from build123d import *

# Parameters (mm, degrees)
SKETCH1_R                      = 15.35
BOSS_EXTRUDE1_DEPTH            = 2.71
SKETCH2_R                      = 2.685
BOSS_EXTRUDE2_DEPTH            = 1.2
DOME1_FACE_RADIUS              = 2.685
DOME1_HEIGHT                   = 0.6
CIRPATTERN1_COUNT              = 3
CIRPATTERN1_COPY_1_FACE_RADIUS = 2.685
CIRPATTERN1_COPY_1_HEIGHT      = 0.6
CIRPATTERN1_COPY_2_FACE_RADIUS = 2.685
CIRPATTERN1_COPY_2_HEIGHT      = 0.6
BOSS_EXTRUDE3_START            = 2.55
SKETCH3_W                      = 5.5
SKETCH3_H                      = 4.2
SKETCH3_W_2                    = 1.5
SKETCH3_H_2                    = 2.8
BOSS_EXTRUDE3_DEPTH            = 2.55
SKETCH4_W                      = 5.5
SKETCH4_H                      = 4.2
BOSS_EXTRUDE4_DEPTH            = 1.44
CHIP_DEPTH                     = 1.7018


with BuildPart() as part:
    # Sketch1 → Boss-Extrude1 (new body)
    with BuildSketch(Plane(origin=(0, 0, 0), x_dir=(1, 0, 0), z_dir=(0, 1, 0))):
        with Locations(Location((0, 0, 0), (0, 0, 270))):
            Circle(SKETCH1_R)
    extrude(amount=BOSS_EXTRUDE1_DEPTH)

    # Sketch2 → Boss-Extrude2 (add)
    with BuildSketch(Plane(origin=(0, 2.71, 0), x_dir=(-1, 0, 0), z_dir=(0, 1, 0))):
        with Locations(Location((-5.5, 9.526279442, 0), (0, 0, 90))):
            Circle(SKETCH2_R)
    boss_extrude2 = extrude(amount=BOSS_EXTRUDE2_DEPTH)

    # Dome1: a dome of height H over a round flat face of radius A is a cap of a sphere of radius (A * A + H * H) / (2 * H)
    dome1_r = (DOME1_FACE_RADIUS * DOME1_FACE_RADIUS + DOME1_HEIGHT * DOME1_HEIGHT) / (2 * DOME1_HEIGHT)
    dome1_base = Plane((5.5, 3.91, 9.526279442), z_dir=(0, 1, 0))
    with Locations(dome1_base.offset(DOME1_HEIGHT - dome1_r)):
        dome1_ball = Sphere(dome1_r, mode=Mode.PRIVATE)
    add(split(dome1_ball, bisect_by=dome1_base, keep=Keep.TOP, mode=Mode.PRIVATE))

    # CirPattern1: Boss-Extrude2 ×3 about axis
    cirpattern1_axis = Axis((0, 0, 0), (0, 1, 0))
    for i in range(1, CIRPATTERN1_COUNT):
        add(boss_extrude2.rotate(cirpattern1_axis, i * 360 / CIRPATTERN1_COUNT))

    # CirPattern1 copy 1: a dome of height H over a round flat face of radius A is a cap of a sphere of radius (A * A + H * H) / (2 * H)
    cirpattern1_copy_1_r = (CIRPATTERN1_COPY_1_FACE_RADIUS * CIRPATTERN1_COPY_1_FACE_RADIUS + CIRPATTERN1_COPY_1_HEIGHT * CIRPATTERN1_COPY_1_HEIGHT) / (2 * CIRPATTERN1_COPY_1_HEIGHT)
    cirpattern1_copy_1_base = Plane((5.5, 3.91, -9.526279442), z_dir=(0, 1, 0))
    with Locations(cirpattern1_copy_1_base.offset(CIRPATTERN1_COPY_1_HEIGHT - cirpattern1_copy_1_r)):
        cirpattern1_copy_1_ball = Sphere(cirpattern1_copy_1_r, mode=Mode.PRIVATE)
    add(split(cirpattern1_copy_1_ball, bisect_by=cirpattern1_copy_1_base, keep=Keep.TOP, mode=Mode.PRIVATE))

    # CirPattern1 copy 2: a dome of height H over a round flat face of radius A is a cap of a sphere of radius (A * A + H * H) / (2 * H)
    cirpattern1_copy_2_r = (CIRPATTERN1_COPY_2_FACE_RADIUS * CIRPATTERN1_COPY_2_FACE_RADIUS + CIRPATTERN1_COPY_2_HEIGHT * CIRPATTERN1_COPY_2_HEIGHT) / (2 * CIRPATTERN1_COPY_2_HEIGHT)
    cirpattern1_copy_2_base = Plane((-11, 3.91, 0), z_dir=(0, 1, 0))
    with Locations(cirpattern1_copy_2_base.offset(CIRPATTERN1_COPY_2_HEIGHT - cirpattern1_copy_2_r)):
        cirpattern1_copy_2_ball = Sphere(cirpattern1_copy_2_r, mode=Mode.PRIVATE)
    add(split(cirpattern1_copy_2_ball, bisect_by=cirpattern1_copy_2_base, keep=Keep.TOP, mode=Mode.PRIVATE))

    # Sketch3 → Boss-Extrude3 (add)
    with BuildSketch(Plane.XZ.offset(BOSS_EXTRUDE3_START)):
        with Locations((0, 13.05)):
            Rectangle(SKETCH3_W, SKETCH3_H)
        with Locations((0, -13.05)):
            Rectangle(SKETCH3_W, SKETCH3_H)
        with Locations((3.5, 13.05)):
            Rectangle(SKETCH3_W_2, SKETCH3_H_2)
        with Locations((-3.5, 13.05)):
            Rectangle(SKETCH3_W_2, SKETCH3_H_2)
        with Locations((3.5, -13.05)):
            Rectangle(SKETCH3_W_2, SKETCH3_H_2)
        with Locations((-3.5, -13.05)):
            Rectangle(SKETCH3_W_2, SKETCH3_H_2)
        with BuildLine():
            Line((2.75, 15.101655538), (2.75, 15.15))
            Line((2.75, 15.15), (2.469817807, 15.15))
            ThreePointArc((2.469817807, 15.15), (2.610020839, 15.126476497), (2.75, 15.101655538))
        make_face()
        with BuildLine():
            ThreePointArc((-2.75, 15.101655538), (-2.610020839, 15.126476497), (-2.469817807, 15.15))
            Line((-2.469817807, 15.15), (-2.75, 15.15))
            Line((-2.75, 15.15), (-2.75, 15.101655538))
        make_face()
        with BuildLine():
            ThreePointArc((-2.469817807, -15.15), (-2.610020839, -15.126476497), (-2.75, -15.101655538))
            Line((-2.75, -15.101655538), (-2.75, -15.15))
            Line((-2.75, -15.15), (-2.469817807, -15.15))
        make_face()
        with BuildLine():
            Line((2.75, -15.15), (2.75, -15.101655538))
            ThreePointArc((2.75, -15.101655538), (2.610020839, -15.126476497), (2.469817807, -15.15))
            Line((2.469817807, -15.15), (2.75, -15.15))
        make_face()
    extrude(amount=-BOSS_EXTRUDE3_DEPTH)

    # Sketch4 → Boss-Extrude4 (add)
    with BuildSketch(Plane.XZ.offset(2.55)):
        Polygon((-2.75, 10.95), (2.75, 10.95), (2.75, 11.65), (2.75, 14.45), (2.75, 15.15), (-2.75, 15.15), (-2.75, 14.45), (-2.75, 11.65), align=None)
        with Locations((0, -13.05)):
            Rectangle(SKETCH4_W, SKETCH4_H)
    extrude(amount=BOSS_EXTRUDE4_DEPTH)

    # Sketch5 → Chip (add)
    with BuildSketch(Plane.XZ):
        Polygon((-5.1644, -9.425953844), (-2.016601499, -2.878979584), (-8.014179317, 0.004667994), (-11.161977818, -6.542306266), align=None)
    extrude(amount=CHIP_DEPTH)


solid = part.part
Geometry check sheet. Reference: the model listing, model coordinates, mm. A direction names the side the tool comes from. Give positions to 0.01 mm unless a question says otherwise; leave off trailing zeros. Order: outer loops, then holes, each group sorted by start corner. A loop starts at its lowest first (then second) coordinate and runs counter-clockwise, first axis right, second up. Notation, with made-up numbers: (24, 82) - (50, 82) arc R6 cw to (50, 89) - close; hole circle Ø8 at (54, -21). An arc over 180 degrees is marked (long way). Answer as a JSON object with one key per item and string values.
(1) Cross-section at B-B (z = -10.5). Record the cut outline in (x, y), then the cut area to 3 significant figures.
Report:
{"outline": "(-11.2, 0) - (11.2, 0) - (11.2, 2.71) - (8, 2.71) - (8, 3.91) arc R6.23 ccw to (3, 3.91) - (3, 2.71) - (-11.2, 2.71) - close", "area": "68.5 mm^2"}
(2) Depth check by flat-ended pin: pin 1 Ø1.3 at (y, z) = (-1.5, -13.5) entering from -X; pin 2 Ø5 at (x, z) = (10.5, 4) entering from -Y; pin 3 Ø1 at (x, z) = (-7.5, -7.5) entering from -Y; pin 4 Ø1.5 at (x, y) = (-2, 3.5) entering from +Z. Enter the tip coordinate at first touch or a pass-through.
Report:
{"pin 1": "x = -4.25", "pin 2": "y = 0", "pin 3": "y = -1.7", "pin 4": "through"}
(3) Cross-section at A-A (x = 0). Record the cut outline in (y, z), then the cut area to 3 significant figures.
Report:
{"outline": "(-3.99, -15.15) - (0, -15.15) - (0, -15.35) - (2.71, -15.35) - (2.71, 15.35) - (0, 15.35) - (0, 15.15) - (-3.99, 15.15) - (-3.99, 10.95) - (0, 10.95) - (0, -10.95) - (-3.99, -10.95) - close", "area": "117 mm^2"}
(4) Material ranges on line 1 (X direction, y = -0.75, z = -12); line 2 (Y direction, x = 8.5, z = -4.5); line 3 (Y direction, x = -6, z = -1.5), recorded low to high.
Report:
{"line 1": "-4.25 to 4.25", "line 2": "0 to 2.71", "line 3": "-1.7 to 2.71"}
(5) Tool access check on faces 4 (the cylindrical face through (2.88, 3.3, 8.94)), 5 (the flat face through (0, -2, 15.15)), 6 (the flat face through (4.25, -1, -13)), 7 (the flat face through (-4, -1, 14.45)), 8 (the flat face through (-4.97, -0.84, -1.46)). Record the directions out of +Z, -Z, +X, -X, +Y, -Y that give a thin tool (end or side, any length) a straight path to the whole face; none if there is none.
Report:
{"face 4": "+Y", "face 5": "+Z, +X, -X, -Y", "face 6": "+Z, -Z, +X, -Y", "face 7": "+Z, -X, -Y", "face 8": "+X, -Y"}
(6) Draft check along Z on faces 1 (the flat face through (-2.75, -3, 13)), 2 (the flat face through (3, -2.55, 13)), 3 (the cylindrical face through (-13.4, 3.3, 1.2)). Enter one of: released by +Z, released by -Z, zero draft, split by the parting line, or undercut.
Report:
{"face 1": "undercut", "face 2": "zero draft", "face 3": "split by the parting line"}
(7) Cross-section at C-C (x = -7). Record the cut outline in (y, z).
Report:
{"outline": "(-1.7, -8.54) - (0, -8.54) - (0, -13.66) - (2.71, -13.66) - (2.71, 13.66) - (0, 13.66) - (0, -0.48) - (-1.7, -0.48) - close"}
(8) Cross-section at D-D (x = 5.5). Record the cut outline in (y, z), then the cut area to 3 significant figures.
Report:
{"outline": "(0, -14.33) - (2.71, -14.33) - (2.71, -12.21) - (3.91, -12.21) arc R6.31 ccw to (3.91, -6.84) - (2.71, -6.84) - (2.71, 6.84) - (3.91, 6.84) arc R6.31 ccw to (3.91, 12.21) - (2.71, 12.21) - (2.71, 14.33) - (0, 14.33) - close", "area": "94.9 mm^2"}
